Part model, mm, in its own coordinate system. Face numbers are marked on the shaded views. A direction names the side the tool comes from. Give positions to 0.01 mm unless a question says otherwise; leave off trailing zeros. Write each loop counter-clockwise with the first axis right and the second up, starting at its lowest first coordinate (ties: lowest second). Pieces come first, ordered by that corner, then holes. Notation, with made-up numbers: (27.5, 83) - (66.5, 83) arc R16 cw to (66.5, 91) - close; hole circle Ø10 at (-11, 26.25). An arc over 180 degrees is marked (long way). Answer in a Markdown table with one row per item. Add a question column.
1. Band-saw the part on A-A on y = 25. Write the cut outline in (x, z).
2. Probe line 1 along Z through (x, y) = (12.5, 27); line 2 along Y through (x, z) = (10.5, -7). List the from-to ranges inside material, lowest first.
3. Band-saw the part on D-D on x = 17.5. Write the cut outline in (y, z).
4. Band-saw the part on B-B on x = 1. Write the cut outline in (y, z), plus the area to 3 significant figures.
5. Drop flat-ended pins along their axis: pin 1 Ø5 at (y, z) = (32.5, 9.5) entering from +X; pin 2 Ø8 at (x, z) = (7.5, 3) entering from +Y; pin 3 Ø15 at (x, z) = (16, 5.5) entering from +Y; pin 4 Ø1.2 at (x, y) = (4, -1) entering from -Z. Give the stop position or say it passes through.
6. Which spindle directions (+Z, -Z, +X, -X, +Y, -Y) get a long thin tool onto all of the face, cutting with end or side? Do the marked faces 1, 2 and 3. Say none if no direction does.
7. Pull direction X, two halves, no side cores. Call the marked faces 4, 5, 6 and 7: released by +X, released by -X, zero draft, split by the parting line, or undercut.
8. Band-saw the part on C-C on z = 0. State how many separate pieces and enclosed holes the cut face has, plus the area to 3 significant figures.
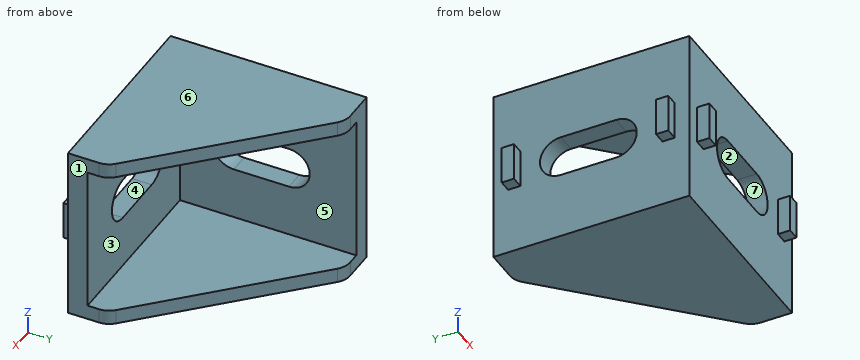
```python
from build123d import *

# Parameters (mm, degrees)
EXTRUDE_1_DEPTH        = 18
EXTRUDE_2_DEPTH        = 3
FILLET_1_R             = 4
FILLET_1_OF_MIRROR_2_R = 4
CUT_EXTRUDE_1_DEPTH    = 5
SKETCH_4_W             = 2.5
SKETCH_4_H             = 7.8
EXTRUDE_3_DEPTH        = 2.5


with BuildPart() as part:
    # Эскиз1 → Бобышка-Вытянуть1 (new body, symmetric)
    with BuildSketch(Plane.XY):
        Polygon((0, 40), (0, 0), (40, 0), (40, 4), (4, 4), (4, 40), align=None)
    extrude(amount=EXTRUDE_1_DEPTH, both=True)

    # Эскиз2 → Бобышка-Вытянуть2 (add)
    with BuildSketch(Plane.XY.offset(18)):
        Polygon((40, 4), (4, 4), (4, 40), (8, 40), (40, 8), align=None)
    extrude_2 = extrude(amount=-EXTRUDE_2_DEPTH)

    # Скругление1
    fillet_1_edges = [part.edges().sort_by_distance(p)[0] for p in [
        (8, 40, 16.5),
        (40, 8, 16.5),
    ]]
    fillet(fillet_1_edges, radius=FILLET_1_R)

    # Зеркальное отражение2: Бобышка-Вытянуть2 across plane
    add(extrude_2.mirror(Plane.XY))

    # Скругление1 of Зеркальное отражение2
    fillet_1_of_mirror_2_edges = [part.edges().sort_by_distance(p)[0] for p in [
        (8, 40, -16.5),
        (40, 8, -16.5),
    ]]
    fillet(fillet_1_of_mirror_2_edges, radius=FILLET_1_OF_MIRROR_2_R)

    # Эскиз3 → Вырез-Вытянуть1 (cut, through all)
    with BuildSketch(Plane(origin=(0, 4, 0), x_dir=(1, 0, 0), z_dir=(0, 1, 0))):
        with BuildLine():
            Line((15, 4.25), (26.25, 4.25))
            ThreePointArc((26.25, 4.25), (30.5, 0), (26.25, -4.25))
            Line((26.25, -4.25), (15, -4.25))
            ThreePointArc((15, -4.25), (10.75, 0), (15, 4.25))
        make_face()
    cut_extrude_1 = extrude(amount=-CUT_EXTRUDE_1_DEPTH, mode=Mode.SUBTRACT)

    # Эскиз4 → Бобышка-Вытянуть3 (add)
    with BuildSketch(Plane.XZ):
        with Locations((4.25, 0)):
            Rectangle(SKETCH_4_W, SKETCH_4_H)
        with Locations((35.75, 0)):
            Rectangle(SKETCH_4_W, SKETCH_4_H)
    extrude_3 = extrude(amount=EXTRUDE_3_DEPTH)

    # Зеркальное отражение3: Вырез-Вытянуть1, Бобышка-Вытянуть3 across plane
    add(cut_extrude_1.mirror(Plane(origin=(0, 0, 0), x_dir=(0, 0, 1), z_dir=(-0.707106781, 0.707106781, 0))), mode=Mode.SUBTRACT)
    add(extrude_3.mirror(Plane(origin=(0, 0, 0), x_dir=(0, 0, 1), z_dir=(-0.707106781, 0.707106781, 0))))


solid = part.part
```
Values:
| question | item | result |
|---|---|---|
| 1 | outline | (0, -18) - (23, -18) - (23, -15) - (4, -15) - (4, -4.25) - (0, -4.25) - close; (0, 4.25) - (4, 4.25) - (4, 15) - (23, 15) - (23, 18) - (0, 18) - close |
| 2 | line 1 | z = -18 to -15, 15 to 18 |
| 2 | line 2 | y = 0 to 4 |
| 3 | outline | (0, -18) - (30.5, -18) - (30.5, -15) - (4, -15) - (4, -4.25) - (0, -4.25) - close; (0, 4.25) - (4, 4.25) - (4, 15) - (30.5, 15) - (30.5, 18) - (0, 18) - close |
| 4 | outline | (0, -18) - (40, -18) - (40, 18) - (0, 18) - close; hole (15, -4.25) - (26.25, -4.25) arc R4.25 ccw to (26.25, 4.25) - (15, 4.25) arc R4.25 ccw to start |
| 4 | area | 1,290 mm² |
| 5 | pin 1 | stops at x = 4 |
| 5 | pin 2 | stops at y = 40 |
| 5 | pin 3 | stops at y = 4 |
| 5 | pin 4 | stops at z = -3.9 |
| 6 | face 1 | +Z, -Z, +X, +Y, -Y |
| 6 | face 2 | +Y, -Y |
| 6 | face 3 | +X, +Y |
| 7 | face 4 | undercut |
| 7 | face 5 | released by +X |
| 7 | face 6 | zero draft |
| 7 | face 7 | undercut |
| 8 | separate pieces | 3 |
| 8 | enclosed holes | 0 |
| 8 | area | 171 mm² |
